Geometry: see drawing. Coordinates: mm, zero at the bounding-box minimum. A direction names the side the tool comes from. Give positions to 0.01 mm unless a question says otherwise; leave off trailing zeros. Write each loop counter-clockwise with the first axis right and the second up, starting at its lowest first coordinate (ties: lowest second). Pieces come first, ordered by that corner, then holes.
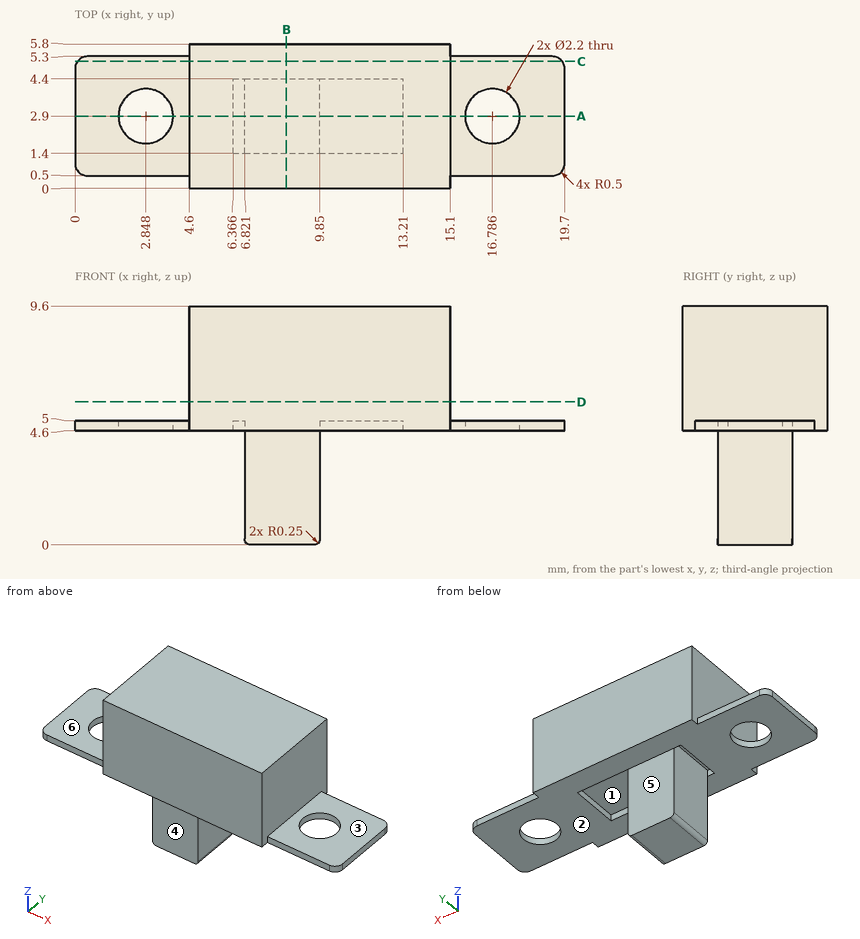
1. Access query for the marked faces 3, 4, 5 and 6. Directions: +Z, -Z, +X, -X, +Y, -Y. A direction counts if a zero-diameter tool reaches every point of the face in a straight line with its end or side. Return the directions, or none.
2. Section query B-B (x = 8.5). Return loops of the section in (y, z), plus the area to 3 significant figures.
3. Section query D-D (z = 5.75). Return loops of the section in (x, y), plus the area to 3 significant figures.
4. Section query A-A (y = 2.9). Return loops of the section in (x, z), plus the area to 3 significant figures.
5. Pull-direction query (X, two-part tool) for the marked faces 1 and 2; classes: pulls with the +X half, pulls with the -X half, needs draft (parallel to the pull), parting line crosses it, or undercut.
6. Pin query (flat end, axial travel): P1, Ø1.5, axis at x = 9, z = 2.5, coming from the -Y side; P2, Ø3, axis at x = 16.79, y = 2.9, coming from the -Z side; P3, Ø2.5, axis at y = 1.5, z = 8.5, coming from the +X side. Return the tip coordinate at first contact, or that it passes through.
7. Section query C-C (y = 5.1). Return loops of the section in (x, z), plus the area to 3 significant figures.
8. Line query: probe 1 along Z at (x, y) = (17.5, 4.2); probe 2 along X at (y, z) = (3.8, 2); probe 3 along X at (y, z) = (3.1, 7.5). Output: solid intervals per line, ascending.
The answers:
1. face 3: +Z, +X, +Y, -Y
1. face 4: -Z, +X, -X, -Y
1. face 5: -Z, +X, -X, +Y
1. face 6: +Z, -X, +Y, -Y
2. outline: (0, 4.6) - (1.4, 4.6) - (1.4, 0) - (4.4, 0) - (4.4, 4.6) - (5.8, 4.6) - (5.8, 9.6) - (0, 9.6) - close
2. area: 42.8 mm2
3. outline: (4.6, 0) - (15.1, 0) - (15.1, 5.8) - (4.6, 5.8) - close
3. area: 60.9 mm2
4. outline: (0, 4.6) - (1.75, 4.6) - (1.75, 5) - (0, 5) - close; (3.95, 4.6) - (6.37, 4.6) - (6.37, 5) - (6.82, 5) - (6.82, 0.25) arc R0.25 ccw to (7.07, 0) - (9.6, 0) arc R0.25 ccw to (9.85, 0.25) - (9.85, 5) - (13.21, 5) - (13.21, 4.6) - (15.69, 4.6) - (15.69, 5) - (15.1, 5) - (15.1, 9.6) - (4.6, 9.6) - (4.6, 5) - (3.95, 5) - close; (17.89, 4.6) - (19.7, 4.6) - (19.7, 5) - (17.89, 5) - close
4. area: 66.8 mm2
5. face 1: undercut
5. face 2: needs draft
6. P1: stops at y = 1.4
6. P2: stops at z = 4.6
6. P3: stops at x = 15.1
7. outline: (0.1, 4.6) - (19.6, 4.6) - (19.6, 5) - (15.1, 5) - (15.1, 9.6) - (4.6, 9.6) - (4.6, 5) - (0.1, 5) - close
7. area: 56.1 mm2
8. probe 1: z = 4.6 to 5
8. probe 2: x = 6.82 to 9.85
8. probe 3: x = 4.6 to 15.1
